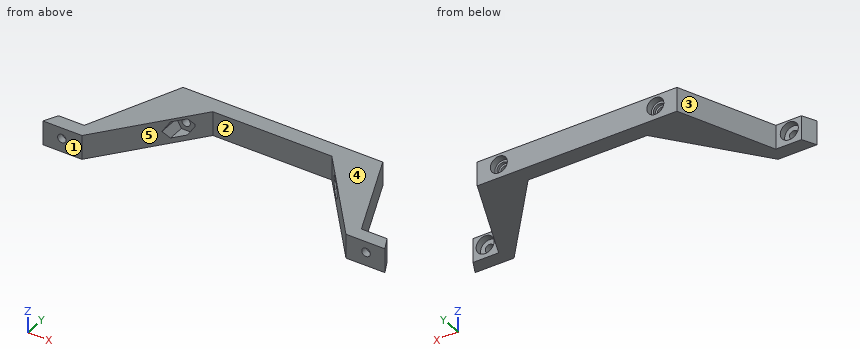
from build123d import *

# Parameters (mm, degrees)
EXTRUDE_1_DEPTH      = 10
SKETCH_7_R           = 1.55
CUT_EXTRUDE_1_DEPTH  = 36.544157215
CUT_EXTRUDE_2_DEPTH  = 8.5
SKETCH_14_R          = 1.575
CUT_EXTRUDE_10_DEPTH = 10
SKETCH_15_R          = 3.35
CUT_EXTRUDE_11_DEPTH = 2.5
SKETCH_19_W          = 126.714157214
SKETCH_19_H          = 0.99604336
CUT_EXTRUDE_14_DEPTH = 40.044157215


with BuildPart() as part:
    # 草图1 → 凸台-拉伸1 (new body)
    with BuildSketch(Plane.XY):
        Polygon((-3.188712924, 13.052848472), (33.811287076, 13.052848472), (33.811287076, 7.052848472), (15.60198174, 7.052848472), (11.74198174, 7.052848472), (-15.114428715, -25.991308743), (-17.614428715, -25.991308743), (-29.545791531, -25.991308743), (-27.045791531, -20.991308743), (-17.548712924, -20.991308743), align=None)
    extrude_1 = extrude(amount=EXTRUDE_1_DEPTH)

    # 镜向1: 凸台-拉伸1 across plane
    add(extrude_1.mirror(Plane(origin=(33.811287076, 13.052848472, 10), x_dir=(0, 0, 1), z_dir=(-1, 0, 0))))

    # 草图5 → 切除-旋转7 (revolve, cut)
    with BuildSketch(Plane.XY.offset(5)):
        Polygon((7.961287076, 13.052848472), (7.961287076, 10.552848472), (7.161287076, 10.552848472), (7.161287076, 9.552848472), (6.361287076, 9.552848472), (4.811287076, 9.552848472), (4.811287076, 13.052848472), align=None)
    cut_revolve_7 = revolve(axis=Axis((4.811287076, 9.552848472, 5), (0, 1, 0)), mode=Mode.SUBTRACT)

    # 草图7 → 切除-拉伸1 (cut, through all)
    with BuildSketch(Plane(origin=(0, 9.552848472, 0), x_dir=(1, 0, 0), z_dir=(0, 1, 0))):
        with Locations((4.811287076, -5)):
            Circle(SKETCH_7_R)
    cut_extrude_1 = extrude(amount=-CUT_EXTRUDE_1_DEPTH, mode=Mode.SUBTRACT)

    # 草图8 → 切除-拉伸2 (cut)
    with BuildSketch(Plane(origin=(0, -5.947151528, 0), x_dir=(1, 0, 0), z_dir=(0, 1, 0))):
        Polygon((8.333123718, -5), (6.572205397, -1.95), (3.050368755, -1.95), (1.289450434, -5), (3.050368755, -8.05), (6.572205397, -8.05), align=None)
    cut_extrude_2 = extrude(amount=CUT_EXTRUDE_2_DEPTH, mode=Mode.SUBTRACT)

    # 草图14 → 切除-拉伸10 (cut)
    with BuildSketch(Plane(origin=(0, -20.991308743, 0), x_dir=(1, 0, 0), z_dir=(0, 1, 0))):
        with Locations((-22.548712924, -5)):
            Circle(SKETCH_14_R)
    cut_extrude_10 = extrude(amount=-CUT_EXTRUDE_10_DEPTH, mode=Mode.SUBTRACT)

    # 草图15 → 切除-拉伸11 (cut)
    with BuildSketch(Plane(origin=(0, -20.991308743, 0), x_dir=(1, 0, 0), z_dir=(0, 1, 0))):
        with Locations((-22.548712924, -5)):
            Circle(SKETCH_15_R)
    cut_extrude_11 = extrude(amount=-CUT_EXTRUDE_11_DEPTH, mode=Mode.SUBTRACT)

    # 镜向3: 切除-旋转7, 切除-拉伸1, 切除-拉伸2, 切除-拉伸10, 切除-拉伸11 across plane
    add(cut_revolve_7.mirror(Plane(origin=(33.811287076, 0, 0), x_dir=(0, 0, 1), z_dir=(1, 0, 0))), mode=Mode.SUBTRACT)
    add(cut_extrude_1.mirror(Plane(origin=(33.811287076, 0, 0), x_dir=(0, 0, 1), z_dir=(1, 0, 0))), mode=Mode.SUBTRACT)
    add(cut_extrude_2.mirror(Plane(origin=(33.811287076, 0, 0), x_dir=(0, 0, 1), z_dir=(1, 0, 0))), mode=Mode.SUBTRACT)
    add(cut_extrude_10.mirror(Plane(origin=(33.811287076, 0, 0), x_dir=(0, 0, 1), z_dir=(1, 0, 0))), mode=Mode.SUBTRACT)
    add(cut_extrude_11.mirror(Plane(origin=(33.811287076, 0, 0), x_dir=(0, 0, 1), z_dir=(1, 0, 0))), mode=Mode.SUBTRACT)

    # 草图19 → 切除-拉伸14 (cut, through all)
    with BuildSketch(Plane(origin=(0, 13.052848472, 0), x_dir=(1, 0, 0), z_dir=(0, 1, 0))):
        with Locations((33.811287076, -9.50197832)):
            Rectangle(SKETCH_19_W, SKETCH_19_H)
    extrude(amount=-CUT_EXTRUDE_14_DEPTH, mode=Mode.SUBTRACT)


solid = part.part
Design review of the part built by this model. Coordinates are the model's own, in mm. Face numbers are marked on the shaded views. A direction names the side the tool comes from. Coordinates: 2 decimals unless noted, no trailing zeros. Write each loop counter-clockwise with the first axis right and the second up, starting at its lowest first coordinate (ties: lowest second). Pieces come first, ordered by that corner, then holes. Notation, with made-up numbers: (42.5, -17) - (76.5, -17) arc R14 ccw to (76.5, 3) - close; hole circle Ø8 at (-24.75, -27). An arc over 180 degrees is marked (long way). One line per item, written item: value.
1) Insertion check: pin 1 (3 mm diameter, centred on x = 62, y = -1, fed in from -Z); pin 2 (1 mm diameter, centred on y = 7, z = 3.5, fed in from -X); pin 3 (5 mm diameter, centred on x = 62.81, z = 5, fed in from -Y); pin 4 (3 mm diameter, centred on y = 0, z = 2.5, fed in from +X). Each pin has a flat end and moves straight along its axis. Give the tip position at first contact, or say it passes through.
Answer sheet:
pin 1: stops at z = 0
pin 2: stops at x = -5.95
pin 3: stops at y = 2.55
pin 4: stops at x = 76.95
2) Mouldability with a two-part tool opening along X and no side actions: class the marked faces 1, 2 and 3 as +X half, -X half, draft (parallel to the pull), parting line (faces both ways), or undercut.
Answer sheet:
face 1: draft
face 2: undercut
face 3: -X half
3) To check wall thickness, follow probe 1 along X at (y, z) = (-23, 3.75); probe 2 along X at (y, z) = (5.5, 4.5); probe 3 along X at (y, z) = (11.7, 5). State the ranges of each line that lie inside material, in increasing order.
Answer sheet:
probe 1: x = -28.05 to -25.66, -19.44 to -12.68, 80.31 to 87.06, 93.28 to 95.67
probe 2: x = -6.37 to 3.34, 6.28 to 10.48, 57.14 to 61.34, 64.28 to 74
probe 3: x = -3.76 to 1.66, 7.96 to 59.66, 65.96 to 71.38
4) Add section A-A (x = 47.5). State the section outline as (y, z) points, plus the area to 3 significant figures.
Answer sheet:
outline: (7.05, 0) - (13.05, 0) - (13.05, 9) - (7.05, 9) - close
area: 54.0 mm2
5) For the marked faces 4 and 5, list the 3-axis set-ups (+Z, -Z, +X, -X, +Y, -Y) from which the entire face can be reached by the end or side of a thin tool; tool diameter is ignored.
Answer sheet:
face 4: +Z, +X, -X, +Y, -Y
face 5: +Z, -Z, -Y
